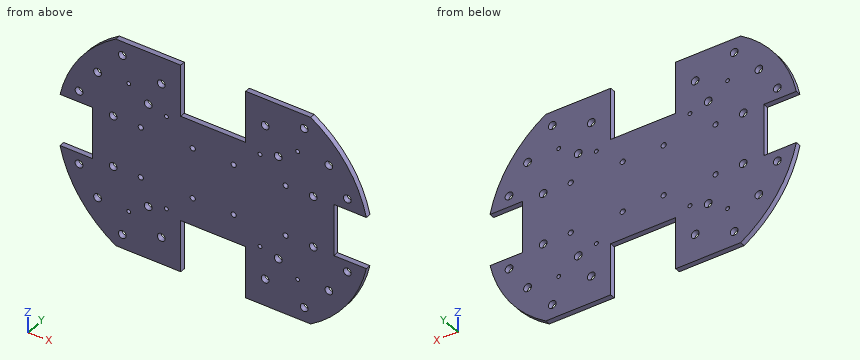
Autodesk Inventor part; units mm, degrees
ref_plane "YZ Plane" through (0, 0, 0) normal (1, 0, 0) x (0, 1, 0)
ref_plane "XZ Plane" through (0, 0, 0) normal (0, 1, 0) x (-1, 0, 0)
ref_plane "XY Plane" through (0, 0, 0) normal (0, 0, 1) x (1, 0, 0)
sketch "Esquisse1" plane through (0, 0, 0) normal (0, 1, 0) x (-1, 0, 0)
  circle A0 centre (0, 0) radius 25 construction
  line L0 (-25, 0) -> (25, 0) construction
  arc A1 (-75, -80.7775) -> (-75, 80.7775) centre (-25, 0) ccw construction
  arc A2 (75, 80.7775) -> (75, -80.7775) centre (25, 0) ccw construction
  line L1 (0, 25) -> (0, 0) construction
  line L2 (-75, 80.7775) -> (75, 80.7775)
  line L3 (-75, -80.7775) -> (75, -80.7775)
  arc A3 (75, -80.7775) -> (75, 80.7775) centre (25, 0) ccw
  arc A4 (-75, 80.7775) -> (-75, -80.7775) centre (-25, 0) ccw
  dimension "d0" = 50
  dimension "d1" = 190
  dimension "d2" = 150
extrude "Extrusion1" add sketch "Esquisse1" along normal blind 4
sketch "Esquisse4" plane through (0, 0, 0) normal (0, -1, 0) x (1, 0, 0)
  line L0 (-50, 40) -> (50, 40) construction
  line L1 (50, 40) -> (50, -40) construction
  line L2 (50, -40) -> (-50, -40) construction
  line L3 (-50, -40) -> (-50, 40) construction
  circle A0 centre (-50, 40) radius 3
  circle A1 centre (50, 40) radius 3
  circle A2 centre (50, -40) radius 3
  circle A3 centre (-50, -40) radius 3
  line L4 (75, 80.7775) -> (-75, 80.7775)
  point P0 (0, 0)
  dimension "d15" = 80
  dimension "d16" = 100
  dimension "d17" = 50
  dimension "d18" = 40
  dimension "d19" = 6
  dimension "d20" = 6
  dimension "d21" = 6
  dimension "d22" = 6
  dimension "d25" = 40.7775
extrude "Extrusion4" cut sketch "Esquisse4" against normal through all
sketch "Esquisse8" plane through (0, 0, 0) normal (0, -1, 0) x (1, 0, 0)
  line L0 (96.5, 35) -> (96.5, -35)
  line L1 (82, 42) -> (96, 42)
  line L2 (96, 42) -> (96, -42)
  line L3 (96, -42) -> (82, -42)
  line L4 (82, -42) -> (82, 42)
  line L5 (96, 21.5) -> (108.5, 21.5)
  line L6 (108.5, 21.5) -> (108.5, -21.5)
  line L7 (108.5, -21.5) -> (96, -21.5)
  line L8 (96, -21.5) -> (96, 21.5)
  line L9 (82, -14.7) -> (76.3, -14.7)
  line L10 (76.3, -14.7) -> (76.3, 14.7)
  line L11 (76.3, 14.7) -> (82, 14.7)
  line L12 (82, 14.7) -> (82, -14.7)
  line L13 (82, 14.7) -> (72, 14.7)
  line L14 (72, 14.7) -> (72, 24.7)
  line L15 (72, 24.7) -> (82, 24.7)
  line L16 (82, 24.7) -> (82, 14.7)
  line L17 (96, 21.5) -> (110.5, 21.5)
  line L18 (110.5, 21.5) -> (110.5, 35.5)
  line L19 (110.5, 35.5) -> (96, 35.5)
  line L20 (96, 35.5) -> (96, 21.5)
  line L21 (96, 42) -> (82, 42)
  line L22 (82, 42) -> (82, 56)
  line L23 (82, 56) -> (96, 56)
  line L24 (96, 56) -> (96, 42)
  line L25 (72, 24.7) -> (82, 14.7) construction
  line L26 (82, 24.7) -> (72, 14.7) construction
  line L27 (110.5, 21.5) -> (96, 35.5) construction
  line L28 (96, 21.5) -> (110.5, 35.5) construction
  line L29 (82, 56) -> (96, 42) construction
  line L30 (82, 42) -> (96, 56) construction
  circle A0 centre (89, 49) radius 3
  circle A1 centre (77, 19.7) radius 3
  circle A2 centre (103.25, 28.5) radius 3
  arc A3 (75, -80.7775) -> (75, 80.7775) centre (25, 0) ccw
  line L31 (108.5, 21.5) -> (115, 21.5)
  line L32 (115, 21.5) -> (115, -21.5)
  line L33 (115, -21.5) -> (108.5, -21.5)
  line L34 (108.5, -21.5) -> (108.5, 21.5)
  line L35 (0, 0) -> (120, 0)
  dimension "d59" = 84
  dimension "d60" = 14
  dimension "d61" = 29.4
  dimension "d62" = 5.7
  dimension "d63" = 12.5
  dimension "d64" = 43
  dimension "d65" = 42
  dimension "d66" = 14.7
  dimension "d67" = 21.5
  dimension "d68" = 14
  dimension "d69" = 14
  dimension "d70" = 14
  dimension "d71" = 10
  dimension "d72" = 10
  dimension "d73" = 6
  dimension "d74" = 6
  dimension "d75" = 6
  dimension "d78" = 6.5
  dimension "d79" = 5
extrude "Extrusion6" cut sketch "Esquisse8" against normal through all contours A0 | A1 | A2
mirror "Symétrie2" about plane through (0, 0, 0) normal (0, 0, 1) of "Extrusion6"
mirror "Symétrie3" about plane through (0, 0, 0) normal (1, 0, 0) of "Extrusion6", "Symétrie2"
sketch "Esquisse11" plane through (0, 4, 0) normal (0, 1, 0) x (1, 0, 0)
  line L0 (15.75, 19.5) -> (55.75, 19.5)
  line L1 (55.75, 19.5) -> (55.75, -19.5)
  line L2 (55.75, -19.5) -> (15.75, -19.5)
  line L3 (15.75, -19.5) -> (15.75, 19.5)
  line L4 (11.75, 23.5) -> (59.75, 23.5)
  line L5 (59.75, 23.5) -> (59.75, -23.5)
  line L6 (59.75, -23.5) -> (11.75, -23.5)
  line L7 (11.75, -23.5) -> (11.75, 23.5)
  point P0 (0, 0)
  dimension "d103" = 40
  dimension "d104" = 48
  dimension "d105" = 4
  dimension "d106" = 47
  dimension "d107" = 39
  dimension "d108" = 4
  dimension "d109" = 23.5
  dimension "d110" = 11.75
hole "Perçage1" at (15.75, 4, -19.5) at (55.75, 4, -19.5) at (55.75, 4, 19.5) at (15.75, 4, 19.5) direction (0, -1, 0) diameter 4 end through all
mirror "Symétrie7" about plane through (0, 0, 0) normal (1, 0, 0) of "Perçage1"
sketch "Esquisse12" plane through (0, 4, 0) normal (0, 1, 0) x (1, 0, 0)
  arc A0 (75, -80.7775) -> (75, 80.7775) centre (25, 0) ccw
  line L0 (92.8709, 20) -> (117.8709, 20)
  line L1 (117.8709, 20) -> (117.8709, -20)
  line L2 (117.8709, -20) -> (92.8709, -20)
  line L3 (92.8709, -20) -> (92.8709, 20)
  arc A1 (117.8709, 20) -> (117.8709, -20) centre (25, 0) ccw
  arc A2 (117.8709, -20) -> (117.8709, 20) centre (25, 0) ccw
  point P0 (0, 0)
  dimension "d111" = 25
  dimension "d112" = 40
extrude "Extrusion9" cut sketch "Esquisse12" against normal through all contours L1 A0 | L2 L3 L0 L1
mirror "Symétrie8" about plane through (0, 0, 0) normal (1, 0, 0) of "Extrusion9"
sketch "Esquisse14" plane through (0, 0, 0) normal (0, -1, 0) x (1, 0, 0)
  line L0 (75, 80.7775) -> (-75, 80.7775)
  line L1 (-25, 80.7775) -> (25, 80.7775)
  line L2 (25, 80.7775) -> (25, 40.7775)
  line L3 (25, 40.7775) -> (-25, 40.7775)
  line L4 (-25, 40.7775) -> (-25, 80.7775)
  point P0 (0, 0)
  dimension "d131" = 50
  dimension "d132" = 25
  dimension "d133" = 40
extrude "Extrusion11" cut sketch "Esquisse14" against normal through all
mirror "Symétrie10" about plane through (0, 0, 0) normal (0, 0, 1) of "Extrusion11"
sketch "Esquisse15" plane through (0, 0, 0) normal (0, -1, 0) x (1, 0, 0)
  line L0 (-40, 60) -> (40, 60) construction
  line L1 (40, 60) -> (40, -60) construction
  line L2 (40, -60) -> (-40, -60) construction
  line L3 (-40, -60) -> (-40, 60) construction
  circle A0 centre (40, 60) radius 3
  circle A1 centre (-40, 60) radius 3
  circle A2 centre (-40, -60) radius 3
  circle A3 centre (40, -60) radius 3
  point P0 (0, 0)
  dimension "d136" = 120
  dimension "d137" = 80
  dimension "d138" = 40
  dimension "d139" = 60
  dimension "d140" = 6
  dimension "d141" = 6
  dimension "d142" = 6
  dimension "d143" = 6
extrude "Extrusion12" cut sketch "Esquisse15" against normal through all
sketch "Esquisse16" plane through (0, 0, 0) normal (0, -1, 0) x (1, 0, 0)
  line L0 (-70, 70) -> (70, 70) construction
  line L1 (70, 70) -> (70, -70) construction
  line L2 (70, -70) -> (-70, -70) construction
  line L3 (-70, -70) -> (-70, 70) construction
  circle A0 centre (70, 70) radius 3
  circle A1 centre (-70, 70) radius 3
  circle A2 centre (-70, -70) radius 3
  circle A3 centre (70, -70) radius 3
  point P0 (0, 0)
  dimension "d146" = 140
  dimension "d147" = 140
  dimension "d148" = 6
  dimension "d149" = 6
  dimension "d150" = 6
  dimension "d151" = 6
  dimension "d152" = 70
  dimension "d153" = 70
extrude "Extrusion13" cut sketch "Esquisse16" against normal through all
sketch "Esquisse17" plane through (0, 0, 0) normal (0, -1, 0) x (1, 0, 0)
  line L0 (-36, 36) -> (36, 36) construction
  line L1 (36, 36) -> (36, -36) construction
  line L2 (36, -36) -> (-36, -36) construction
  line L3 (-36, -36) -> (-36, 36) construction
  circle A0 centre (-36, 36) radius 1.5
  circle A1 centre (36, 36) radius 1.5
  circle A2 centre (36, -36) radius 1.5
  circle A3 centre (-36, -36) radius 1.5
  point P0 (0, 0)
  dimension "d156" = 72
  dimension "d157" = 72
  dimension "d158" = 3
  dimension "d159" = 3
  dimension "d160" = 3
  dimension "d161" = 3
  dimension "d162" = 36
  dimension "d163" = 36
extrude "Extrusion14" cut sketch "Esquisse17" against normal through all
sketch "Esquisse18" plane through (0, 0, 0) normal (0, -1, 0) x (1, 0, 0)
  line L0 (-65, 50) -> (65, 50) construction
  line L1 (65, 50) -> (65, -50) construction
  line L2 (65, -50) -> (-65, -50) construction
  line L3 (-65, -50) -> (-65, 50) construction
  circle A0 centre (-65, 50) radius 1.5
  circle A1 centre (65, 50) radius 1.5
  circle A2 centre (65, -50) radius 1.5
  circle A3 centre (-65, -50) radius 1.5
  point P0 (0, 0)
  dimension "d166" = 3
  dimension "d167" = 3
  dimension "d168" = 3
  dimension "d169" = 3
  dimension "d170" = 100
  dimension "d171" = 130
  dimension "d172" = 65
  dimension "d173" = 50
extrude "Extrusion15" cut sketch "Esquisse18" against normal through all
equation "\"d20\" = d19"
equation "\"d21\" = d19"
equation "\"d22\" = d19"
equation "\"d65\" = 0.5 * d59"
equation "\"d66\" = 0.5 * d61"
equation "\"d67\" = 0.5 * d64"
equation "\"d68\" = d60"
equation "\"d70\" = d69"
properties part number "base"
Model file for the job. Use its own axes, mm. Give positions to 0.01 mm unless a question says otherwise; leave off trailing zeros. Loops run counter-clockwise (first coordinate to the right, second up) from the corner with the lowest first, then second, coordinate; pieces in that order, holes last. Notation, with made-up numbers: (-25, 70.5) -> (30, 70.5) arc R7 cw to (30, 74.5) -> close; hole circle Ø10 at (43.25, 11.25). An arc over 180 degrees is marked (long way). Use a Markdown table: item, result. Add a question column.
(1) Slice it at A-A on x = 50. List the corners of the cut face in (y, z).
(2) Drop flat-ended pins along their axis: pin 1 Ø2.5 at (x, z) = (65, -50) entering from -Y; pin 2 Ø8 at (x, z) = (103.25, -28.5) entering from -Y; pin 3 Ø1.2 at (y, z) = (1, -51.5) entering from -X. Give the stop position or say it passes through.
(3) Wall check: line 1 along Z through (x, y) = (49.5, 2.75); line 2 along Z through (x, y) = (-36, 1.85); line 3 along X through (y, z) = (1.1, 51). Give the ranges that are in metal, low to high.
(4) Slice it at B-B on z = 28.5. List the corners of the cut face in (x, y), and give its area (3 significant figures).
(5) Slice it at D-D on z = 60. List the corners of the cut face in (x, y).
(6) Slice it at C-C on x = -103.25. List the corners of the cut face in (y, z), and give its area (3 significant figures).
Filled sheet:
| question | item | result |
|---|---|---|
| 1 | outline | (0, -80.78) -> (4, -80.78) -> (4, -43) -> (0, -43) -> close; (0, -37) -> (4, -37) -> (4, 37) -> (0, 37) -> close; (0, 43) -> (4, 43) -> (4, 80.78) -> (0, 80.78) -> close |
| 2 | pin 1 | through |
| 2 | pin 2 | y = 0 |
| 2 | pin 3 | x = -105.21 |
| 3 | line 1 | -80.78 to -42.96, -37.04 to 37.04, 42.96 to 80.78 |
| 3 | line 2 | -80.78 to -37.5, -34.5 to 34.5, 37.5 to 80.78 |
| 3 | line 3 | -105.15 to -91.24, -86.76 to -66.12, -63.88 to -25, 25 to 63.88, 66.12 to 86.76, 91.24 to 105.15 |
| 4 | outline | (-115.62, 0) -> (-106.25, 0) -> (-106.25, 4) -> (-115.62, 4) -> close; (-100.25, 0) -> (100.25, 0) -> (100.25, 4) -> (-100.25, 4) -> close; (106.25, 0) -> (115.62, 0) -> (115.62, 4) -> (106.25, 4) -> close |
| 4 | area | 877 mm2 |
| 5 | outline | (-98.65, 0) -> (-43, 0) -> (-43, 4) -> (-98.65, 4) -> close; (-37, 0) -> (-25, 0) -> (-25, 4) -> (-37, 4) -> close; (25, 0) -> (37, 0) -> (37, 4) -> (25, 4) -> close; (43, 0) -> (98.65, 0) -> (98.65, 4) -> (43, 4) -> close |
| 6 | outline | (0, -53.87) -> (4, -53.87) -> (4, -31.5) -> (0, -31.5) -> close; (0, -25.5) -> (4, -25.5) -> (4, -20) -> (0, -20) -> close; (0, 20) -> (4, 20) -> (4, 25.5) -> (0, 25.5) -> close; (0, 31.5) -> (4, 31.5) -> (4, 53.87) -> (0, 53.87) -> close |
| 6 | area | 223 mm2 |
